from build123d import *

# Parameters (mm, degrees)
F0_W     = 120
F0_H     = 80
F0_R     = 12.5
F1_DEPTH = 3
F2_R     = 3.5
F3_DEPTH = 18
F4_R     = 0.9
F5_DEPTH = 7


with BuildPart() as f1:
    # F0 (on Top) → F1 (new body)
    with BuildSketch(Plane.XY):
        Rectangle(F0_W, F0_H)
        Circle(F0_R, mode=Mode.SUBTRACT)
    extrude(amount=F1_DEPTH)

    # F2 (on face) → F3 (join)
    with BuildSketch(Plane.XY.offset(3)):
        with Locations((-13, 10)):
            Circle(F2_R)
        with Locations((13, 10)):
            Circle(F2_R)
        with Locations((13, -10)):
            Circle(F2_R)
        with Locations((-13, -10)):
            Circle(F2_R)
    extrude(amount=F3_DEPTH)

    # F4 (on face) → F5 (cut)
    with BuildSketch(Plane.XY.offset(21)):
        with Locations((-13, 10)):
            Circle(F4_R)
        with Locations((13, 10)):
            Circle(F4_R)
        with Locations((13, -10)):
            Circle(F4_R)
        with Locations((-13, -10)):
            Circle(F4_R)
    extrude(amount=-F5_DEPTH, mode=Mode.SUBTRACT)


solid = f1.part
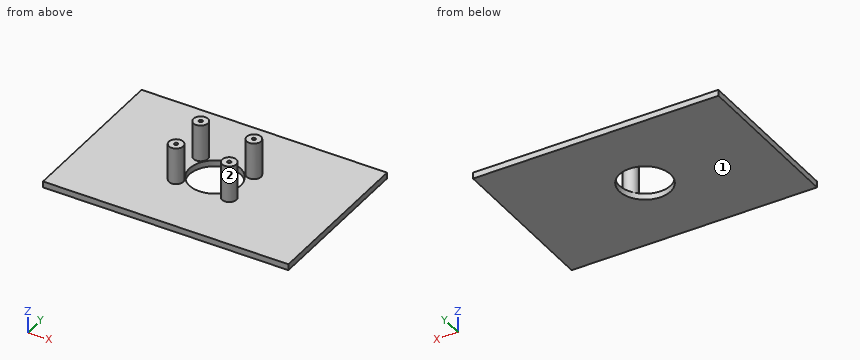
CAD build for the part. Positions are in the model's coordinates, mm. Face numbers are marked on the shaded views. Round coordinates to 2 decimals unless told otherwise and drop trailing zeros. Loops run counter-clockwise (first coordinate to the right, second up) from the corner with the lowest first, then second, coordinate; pieces in that order, holes last. Notation, with made-up numbers: M 50,17 L 92,17 A34 ccw 92,47 Z; hole C 30,65.25 d9. An arc over 180 degrees is marked long. One line per question, with ' | ' between items. Start each with the question number.
Item 1: Wall check: line 1 (Y direction, x = -13, z = 18.75); line 2 (Y direction, x = 0, z = 2.2); line 3 (Z direction, x = 47.5, y = 15). Give the ranges that are in metal, low to high.
Item 2: Pin check, flat tips, straight feed: pin 1 Ø10 at (x, z) = (-48, 10.5) entering from +Y; pin 2 Ø8 at (x, z) = (7.5, 10.5) entering from -Y; pin 3 Ø0.9 at (x, y) = (-13, 10) entering from +Z. Stop position of each tip, or through.
Item 3: Cut at D-D, the plane y = -18. Write the cut outline in (x, z), plus the area to 3 significant figures.
Item 4: Cut at B-B, the plane x = 0. Write the cut outline in (y, z).
Item 5: Cut at C-C, the plane z = 10.75. Write the cut outline in (x, y), plus the area to 3 significant figures.
Item 6: Two-plate mould, pull along Y, no slides. Class the marked faces 1 and 2: pulls with the +Y half, pulls with the -Y half, needs draft (parallel to the pull), parting line crosses it, or undercut.
Item 7: Cut at A-A, the plane z = 16.75. Write the cut outline in (x, y).
Responses:
1) line 1: y = -13.5 to -10.9, -9.1 to -6.5, 6.5 to 9.1, 10.9 to 13.5 | line 2: y = -40 to -12.5, 12.5 to 40 | line 3: z = 0 to 3
2) pin 1: passes through | pin 2: stops at y = -13.16 | pin 3: stops at z = 14
3) outline: M -60,0 L 60,0 L 60,3 L -60,3 Z | area: 360 mm²
4) outline: M -40,0 L -12.5,0 L -12.5,3 L -40,3 Z; M 12.5,0 L 40,0 L 40,3 L 12.5,3 Z
5) outline: C -13,-10 d7; C -13,10 d7; C 13,-10 d7; C 13,10 d7 | area: 154 mm²
6) face 1: needs draft | face 2: undercut
7) outline: C -13,-10 d7; C -13,10 d7; C 13,-10 d7; C 13,10 d7; hole C -13,-10 d1.8; hole C -13,10 d1.8; hole C 13,-10 d1.8; hole C 13,10 d1.8
